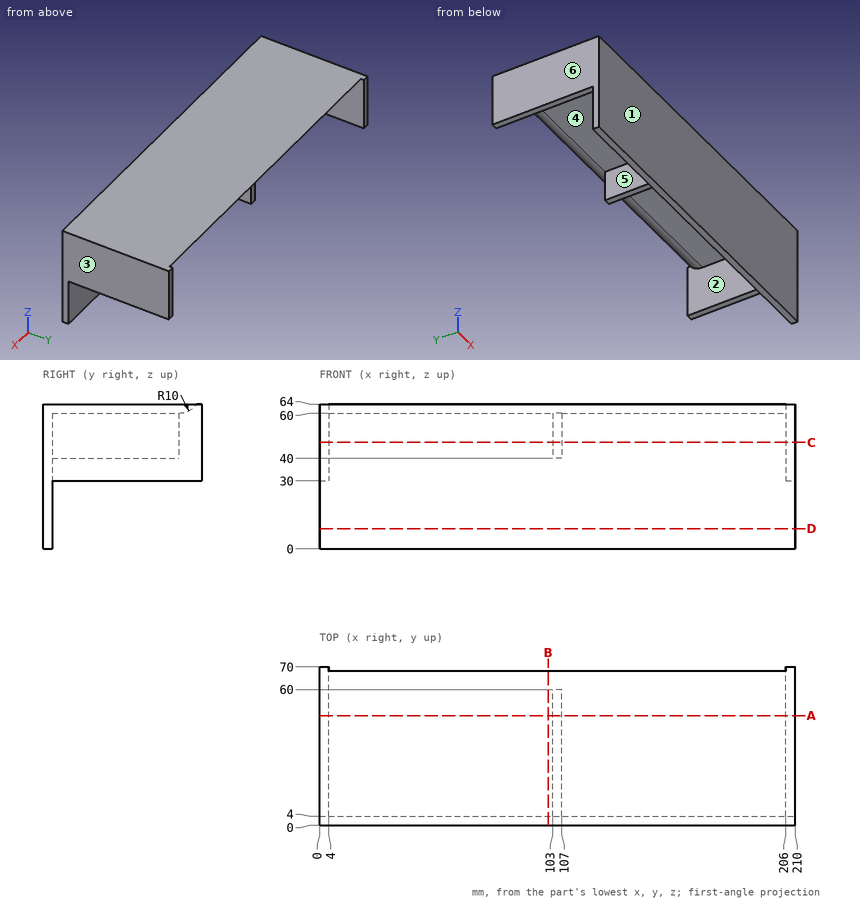
Can you work these out from the drawing? Everything is in mm from the part's minimum corner. A direction names the side the tool comes from. Coordinates: 2 decimals unless noted, no trailing zeros. Write each loop counter-clockwise with the first axis right and the second up, starting at its lowest first coordinate (ties: lowest second). Pieces come first, ordered by that corner, then holes. Notation, with made-up numbers: (78, -31) - (90, -31) arc R37 ccw to (90, 5) - close; hole circle Ø7 at (21, 83). An arc over 180 degrees is marked (long way). Use a Markdown table: item, result.
Q1. I'm going to push flat-ended pins straight in: pin 1 Ø8 at (x, y) = (62, 40) entering from -Z; pin 2 Ø6 at (x, z) = (176, 9) entering from +Y; pin 3 Ø3 at (x, y) = (104, 37) entering from -Z. Where does each tip first touch, or does it pass through?
Geometry check:
| item | result |
|---|---|
| pin 1 | stops at z = 60 |
| pin 2 | stops at y = 4 |
| pin 3 | stops at z = 40 |
Q2. Which directions (+Z, -Z, +X, -X, +Y, -Y) give clear straight access to the entire face, cutting with the end or side of a thin tool? Please do the marked faces 1 and 2.
Geometry check:
| item | result |
|---|---|
| face 1 | +Z, -Z, +X, -X, -Y |
| face 2 | -Z, +Y |
Q3. Thinking about a two-plate mould opening in X: for the marked faces 3, 4, 5 and 6, which applies, +X half, -X half, draft (parallel to the pull), parting line (faces both ways), or undercut?
Geometry check:
| item | result |
|---|---|
| face 3 | +X half |
| face 4 | undercut |
| face 5 | undercut |
| face 6 | -X half |
Q4. Please list where these lines run through material, in increasing order: L1, parallel to X at y = 51.5, z = 55; L2, parallel to Y at x = 55.5, z = 42.5; L3, parallel to Z at x = 149, y = 32.5.
Geometry check:
| item | result |
|---|---|
| L1 | x = 0 to 4, 103 to 107, 206 to 210 |
| L2 | y = 0 to 4 |
| L3 | z = 60 to 64 |
Q5. Imagine slicing it at B-B (x = 101). List the corners of the cut face in (y, z) for me.
Geometry check:
| item | result |
|---|---|
| outline | (0, 0) - (4, 0) - (4, 60) - (60, 60) arc R10 ccw to (68, 64) - (0, 64) - close |
Q6. Imagine slicing it at C-C (z = 47). List the corners of the cut face in (x, y) for me, and give its area (3 significant figures).
Geometry check:
| item | result |
|---|---|
| outline | (0, 0) - (210, 0) - (210, 70) - (206, 70) - (206, 4) - (107, 4) - (107, 60) - (103, 60) - (103, 4) - (4, 4) - (4, 70) - (0, 70) - close |
| area | 1,590 mm2 |
Q7. Imagine slicing it at A-A (y = 48.5). List the corners of the cut face in (x, z) for me, and give its area (3 significant figures).
Geometry check:
| item | result |
|---|---|
| outline | (0, 30) - (4, 30) - (4, 60) - (103, 60) - (103, 40) - (107, 40) - (107, 60) - (206, 60) - (206, 30) - (210, 30) - (210, 64) - (0, 64) - close |
| area | 1,160 mm2 |
Q8. Imagine slicing it at D-D (z = 9). List the corners of the cut face in (x, y) for me.
Geometry check:
| item | result |
|---|---|
| outline | (0, 0) - (210, 0) - (210, 4) - (0, 4) - close |
